Geometry check sheet. Reference: the model listing, model coordinates, mm. A direction names the side the tool comes from. Round coordinates to 2 decimals unless told otherwise and drop trailing zeros. Order: outer loops, then holes, each group sorted by start corner. A loop starts at its lowest first (then second) coordinate and runs counter-clockwise, first axis right, second up. Notation, with made-up numbers: (73, -13) - (125, -13) arc R22 cw to (125, -6) - close; hole circle Ø8 at (15.5, 89.25). An arc over 180 degrees is marked (long way). Return JSON: item names as keys, results as strings. Group by question number.
Q1. Sectioned sample at C-C, the plane z = -52. Record the cut outline in (x, y).
Q2. Tool access check on faces 1 (the cylindrical face through (17, 5, -52)), 2 (the cylindrical face through (41.445, 4.93, 37.979)). Record the directions out of +Z, -Z, +X, -X, +Y, -Y that give a thin tool (end or side, any length) a straight path to the whole face; none if there is none.
Q3. Sectioned sample at B-B, the plane x = 22. Record the cut outline in (y, z).
Q4. Material ranges on line 1 along Z through (x, y) = (-29.5, 0.75); line 2 along Z through (x, y) = (-1.5, 0.5); line 3 along X through (y, z) = (6.5, -52), recorded low to high.
Q5. Gauge pin test, flat ends, axial feed: pin 1 Ø3 at (y, z) = (5, 2.5) entering from -X; pin 2 Ø1.5 at (x, y) = (36.5, 1.5) entering from -Z. Record the tip position at first contact, or that the pin passes through.
Q6. Draft check along Z on faces 3 (the flat face through (-10, 5, -47)), 4 (the cylindrical face through (47.972, 4.93, 45.594)), 5 (the flat face through (51, 0, 4)). Enter one of: pulls with the +Z half, pulls with the -Z half, needs draft (parallel to the pull), parting line crosses it, or undercut.
Q7. Sectioned sample at D-D, the plane x = 55. Record the cut outline in (y, z), then the cut area to 3 significant figures.
Q8. Sectioned sample at A-A, the plane z = -9.5. Record the cut outline in (x, y), then the cut area to 3 significant figures.
```python
from build123d import *

# Parameters (mm, degrees)
SKETCH1_R           = 2
BOSS_EXTRUDE1_DEPTH = 10


with BuildPart() as part:
    # Sketch1 → Boss-Extrude1 (new body)
    with BuildSketch(Plane(origin=(0, 0, 0), x_dir=(1, 0, 0), z_dir=(0, 1, 0))):
        with BuildLine():
            Line((20, -47), (-40, -47))
            Line((-40, -47), (-40, -57))
            Line((-40, -57), (20, -57))
            ThreePointArc((20, -57), (48.284271247, -45.284271247), (60, -17))
            Line((60, -17), (60, 17))
            ThreePointArc((60, 17), (48.284271247, 45.284271247), (20, 57))
            Line((20, 57), (-40, 57))
            Line((-40, 57), (-40, 47))
            Line((-40, 47), (20, 47))
            ThreePointArc((20, 47), (41.213203436, 38.213203436), (50, 17))
            Line((50, 17), (50, -17))
            ThreePointArc((50, -17), (41.213203436, -38.213203436), (20, -47))
        make_face()
        with Locations(Location((55, 9.5, 0), (0, 0, 270))):
            Circle(SKETCH1_R, mode=Mode.SUBTRACT)
        with Locations(Location((55, -9.5, 0), (0, 0, 270))):
            Circle(SKETCH1_R, mode=Mode.SUBTRACT)
        with Locations(Location((15, 52, 0), (0, 0, 270))):
            Circle(SKETCH1_R, mode=Mode.SUBTRACT)
        with Locations(Location((15, -52, 0), (0, 0, 270))):
            Circle(SKETCH1_R, mode=Mode.SUBTRACT)
        with Locations(Location((-18.651513194, 52, 0), (0, 0, 270))):
            Circle(SKETCH1_R, mode=Mode.SUBTRACT)
        with Locations(Location((-31.151513194, 52, 0), (0, 0, 270))):
            Circle(SKETCH1_R, mode=Mode.SUBTRACT)
        with Locations(Location((-18.651513194, -52, 0), (0, 0, 270))):
            Circle(SKETCH1_R, mode=Mode.SUBTRACT)
        with Locations(Location((-31.151513194, -52, 0), (0, 0, 270))):
            Circle(SKETCH1_R, mode=Mode.SUBTRACT)
    extrude(amount=BOSS_EXTRUDE1_DEPTH)


solid = part.part
```
Reply:
{
 "1": {"outline": "(-40, 0) - (-33.15, 0) - (-33.15, 10) - (-40, 10) - close; (-29.15, 0) - (-20.65, 0) - (-20.65, 10) - (-29.15, 10) - close; (-16.65, 0) - (13, 0) - (13, 10) - (-16.65, 10) - close; (17, 0) - (39.36, 0) - (39.36, 10) - (17, 10) - close"},
 "2": {"face 1": "+Y, -Y", "face 2": "-X, +Y, -Y"},
 "3": {"outline": "(0, -56.95) - (10, -56.95) - (10, -46.93) - (0, -46.93) - close; (0, 46.93) - (10, 46.93) - (10, 56.95) - (0, 56.95) - close"},
 "4": {"line 1": "-57 to -53.13, -50.87 to -47, 47 to 50.87, 53.13 to 57", "line 2": "-57 to -47, 47 to 57", "line 3": "-40 to -33.15, -29.15 to -20.65, -16.65 to 13, 17 to 39.36"},
 "5": {"pin 1": "x = 50", "pin 2": "z = -53.77"},
 "6": {"face 3": "undercut", "face 4": "pulls with the +Z half", "face 5": "needs draft"},
 "7": {"outline": "(0, -36.36) - (10, -36.36) - (10, -11.5) - (0, -11.5) - close; (0, -7.5) - (10, -7.5) - (10, 7.5) - (0, 7.5) - close; (0, 11.5) - (10, 11.5) - (10, 36.36) - (0, 36.36) - close", "area": "647 mm^2"},
 "8": {"outline": "(50, 0) - (53, 0) - (53, 10) - (50, 10) - close; (57, 0) - (60, 0) - (60, 10) - (57, 10) - close", "area": "60.0 mm^2"}
}
